Could you check a few things on this model? Use its own coordinates, in mm. Face numbers are marked on the shaded views. Give positions to 0.01 mm unless a question says otherwise; leave off trailing zeros. Loops run counter-clockwise (first coordinate to the right, second up) from the corner with the lowest first, then second, coordinate; pieces in that order, holes last. Notation, with made-up numbers: (39, 50) - (80, 50) arc R30 ccw to (80, 78) - close; hole circle Ø9 at (-3, -14.5). An arc over 180 degrees is marked (long way). Use CSV: the item, a comma, the result in double quotes.
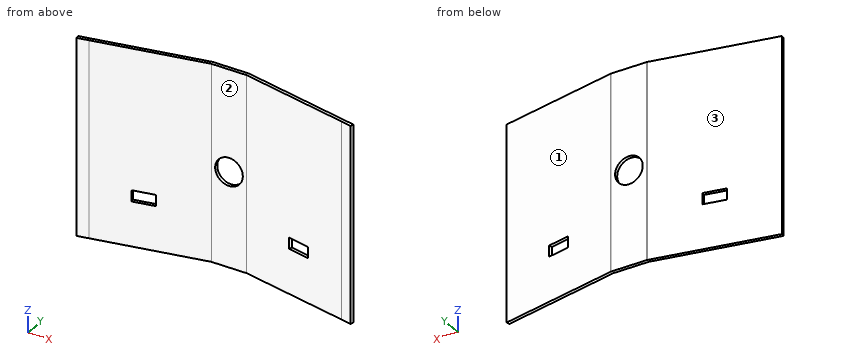
from build123d import *

# Parameters (mm, degrees)
BOSS_EXTRUDE1_DEPTH      = 3
BOSS_EXTRUDE2_DEPTH      = 88
BOSS_EXTRUDE2_DEPTH_BACK = 88
CUT_EXTRUDE1_DEPTH       = 50
SKETCH4_R                = 12.5
CUT_EXTRUDE2_DEPTH       = 25.999792682
SKETCH5_W                = 20
SKETCH5_H                = 10
CUT_EXTRUDE3_DEPTH       = 53.630567568
SKETCH6_W                = 20
SKETCH6_H                = 10
CUT_EXTRUDE4_DEPTH       = 53.630567568


with BuildPart() as part:
    # Sketch1 → Boss-Extrude1 (new body)
    with BuildSketch(Plane.XY):
        Polygon((-16, 19.999811529), (16, 19.999811529), (113.979628183, 0), (113.979628183, -10), (-113.979628183, -10), (-113.979628183, 0), align=None)
    extrude(amount=BOSS_EXTRUDE1_DEPTH)

    # Sketch2 → Boss-Extrude2 (add, two sides)
    with BuildSketch(Plane.XY.offset(3)) as boss_extrude2_sk:
        Polygon((-113.979628183, 0), (-16, 19.999811529), (16, 19.999811529), (113.979628183, 0), (123.777591001, -1.999981153), (124.377585347, 0.939407693), (16.599994346, 22.939200374), (16, 22.999811529), (-16, 22.999811529), (-16.599994346, 22.939200374), (-124.377585347, 0.939407693), (-123.777591001, -1.999981153), align=None)
    extrude(amount=BOSS_EXTRUDE2_DEPTH)
    extrude(boss_extrude2_sk.sketch, amount=-BOSS_EXTRUDE2_DEPTH_BACK)

    # Sketch3 → Cut-Extrude1 (cut)
    with BuildSketch(Plane.XY.offset(3)):
        Polygon((113.979628183, 0), (16, 19.999811529), (-16, 19.999811529), (-113.979628183, 0), (-113.979628183, -10), (113.979628183, -10), align=None)
    extrude(amount=-CUT_EXTRUDE1_DEPTH, mode=Mode.SUBTRACT)

    # Sketch4 → Cut-Extrude2 (cut, through all)
    with BuildSketch(Plane(origin=(0, 22.999811529, 0), x_dir=(1, 0, 0), z_dir=(0, 1, 0))):
        Circle(SKETCH4_R)
    extrude(amount=-CUT_EXTRUDE2_DEPTH, mode=Mode.SUBTRACT)

    # Sketch5 → Cut-Extrude3 (cut, through all)
    with BuildSketch(Plane(origin=(-5.159093546, 25.274541546, 0), x_dir=(0.979796282, 0.199998115, 0), z_dir=(-0.199998115, 0.979796282, 0))):
        with Locations((-66.676815897, 40)):
            Rectangle(SKETCH5_W, SKETCH5_H)
    extrude(amount=-CUT_EXTRUDE3_DEPTH, mode=Mode.SUBTRACT)

    # Sketch6 → Cut-Extrude4 (cut, through all)
    with BuildSketch(Plane(origin=(5.159093546, 25.274541546, 0), x_dir=(0.979796282, -0.199998115, 0), z_dir=(0.199998115, 0.979796282, 0))):
        with Locations((66.676815897, 40)):
            Rectangle(SKETCH6_W, SKETCH6_H)
    extrude(amount=-CUT_EXTRUDE4_DEPTH, mode=Mode.SUBTRACT)


solid = part.part
1) Suppose I cut it at D-D (x = -64). Please give me the cut outline in (y, z), plus the area to 3 significant figures.
Answer below:
outline,"(10.2, -85) - (13.26, -85) - (13.26, -45) - (10.2, -45) - close; (10.2, -35) - (13.26, -35) - (13.26, 91) - (10.2, 91) - close"
area,"508 mm2"
2) Suppose I cut it at C-C (z = -65). Please give me the cut outline in (x, y), plus the area to 3 significant figures.
Answer below:
outline,"(-124.38, 0.94) - (-123.78, -2) - (-16, 20) - (16, 20) - (123.78, -2) - (124.38, 0.94) - (16.6, 22.94) - (16, 23) - (-16, 23) - (-16.6, 22.94) - close"
area,"758 mm2"
3) I'm going to push flat-ended pins straight in: P1, Ø4, axis at x = -67.5, z = 59.5, coming from the +Y side; P2, Ø5, axis at x = -23.5, z = 11, coming from the -Y side; P3, Ø2, axis at x = -97, z = -24, coming from the -Y side; P4, Ø12, axis at x = 34, y = 4.5, coming from the +Z side. Where does each tip first touch, or does it pass through?
Answer below:
P1,"stops at y = 12.96"
P2,"stops at y = 17.96"
P3,"stops at y = 3.26"
P4,"passes through"
4) We'd pull the mould along X, two halves only. Please class the marked faces 1, 2 and 3: +X half, -X half, draft (parallel to the pull), parting line (faces both ways), or undercut.
Answer below:
face 1,"+X half"
face 2,"undercut"
face 3,"-X half"
5) Suppose I cut it at A-A (z = -3.5). Please give me the cut outline in (x, y), plus the area to 3 significant figures.
Answer below:
outline,"(-124.38, 0.94) - (-123.78, -2) - (-16, 20) - (-12, 20) - (-12, 23) - (-16, 23) - (-16.6, 22.94) - close; (12, 20) - (16, 20) - (123.78, -2) - (124.38, 0.94) - (16.6, 22.94) - (16, 23) - (12, 23) - close"
area,"686 mm2"
6) I need wall thicknesses on line 1 along Z through (x, y) = (0, 20.75); line 2 along Y through (x, z) = (4.5, -50); line 3 along Y through (x, z) = (-112.5, 18). Which ranges of each line are inside material? Lowest first, please.
Answer below:
line 1,"z = -85 to -12.5, 12.5 to 91"
line 2,"y = 20 to 23"
line 3,"y = 0.3 to 3.36"
7) Suppose I cut it at B-B (x = 0). Please give me the cut outline in (y, z).
Answer below:
outline,"(20, -85) - (23, -85) - (23, -12.5) - (20, -12.5) - close; (20, 12.5) - (23, 12.5) - (23, 91) - (20, 91) - close"
